from build123d import *

# Parameters (mm, degrees)
PAD_DEPTH       = 25
FILLET_R        = 3
SKETCH009_R     = 7
PAD001_DEPTH    = 6
SKETCH_R        = 12.5
PAD002_DEPTH    = 9.5
POCKET_DEPTH    = 21.498539
SKETCH003_R     = 2.9
POCKET001_DEPTH = 21.498539
POCKET002_DEPTH = 16
POCKET003_DEPTH = 27
SKETCH008_R     = 3.6
POCKET004_DEPTH = 10
SKETCH017_R     = 6.528292
POCKET005_DEPTH = 3
CHAMFER_SIZE    = 2


with BuildPart() as part:
    # Sketch007 → Pad (new body, symmetric)
    with BuildSketch(Plane.XY):
        Polygon((0, 0), (6, 0), (6, 33.225744), (20.888192, 31.397703), (21.497539, 36.360434), (0, 39), align=None)
    extrude(amount=PAD_DEPTH, both=True)

    # Fillet
    fillet_edges = [part.edges().sort_by_distance(p)[0] for p in [
        (0, 39, 0),
        (6, 33.225744, 0),
    ]]
    fillet(fillet_edges, radius=FILLET_R)

    # Sketch009 (on Face7 of Fillet) → Pad001 (join)
    with BuildSketch(Plane(origin=(0, 0, 0), x_dir=(0, -1, 0), z_dir=(-1, 0, 0))):
        with Locations((-7, 25)):
            Circle(SKETCH009_R)
    extrude(amount=-PAD001_DEPTH)

    # Sketch → Pad002 (join)
    with BuildSketch(Plane(origin=(0, 0, 0), x_dir=(0, -1, 0), z_dir=(-1, 0, 0))):
        with BuildLine():
            Line((40.112649, -31.334923), (0, -1.650119))
            Line((0, -1.650119), (-36.144043, -17.199829))
            Line((19.887351, -58.665077), (-36.144043, -17.199829))
            ThreePointArc((19.887351, -58.665077), (43.665077, -55.112649), (40.112649, -31.334923))
        make_face()
        with Locations((30, -45)):
            Circle(SKETCH_R, mode=Mode.SUBTRACT)
    extrude(amount=-PAD002_DEPTH)

    # Sketch013 → Pocket (cut, through all)
    with BuildSketch(Plane(origin=(0, 0, 0), x_dir=(0, -1, 0), z_dir=(-1, 0, 0))):
        Polygon((22.699889, -37.062297), (13.507356, -29.348846), (26.630219, -13.709626), (25.864174, -13.066839), (11.455736, -30.238147), (21.414314, -38.594386), align=None)
    extrude(amount=-POCKET_DEPTH, mode=Mode.SUBTRACT)

    # Sketch003 (on Face19 of Pad002) → Pocket001 (cut, through all)
    with BuildSketch(Plane(origin=(0, 0, 0), x_dir=(0, -1, 0), z_dir=(-1, 0, 0))):
        with Locations((-7, -25)):
            Circle(SKETCH003_R)
        with Locations((-7, 25)):
            Circle(SKETCH003_R)
    extrude(amount=-POCKET001_DEPTH, mode=Mode.SUBTRACT)

    # Sketch015 → Pocket002 (cut)
    with BuildSketch(Plane(origin=(0, 0.311228, -0.406819), x_dir=(1, 0, 0), z_dir=(0, -0.607611, 0.794235))):
        Polygon((4.690891, -37.115485), (6.690891, -35.960785), (6.690891, -33.651383), (4.690891, -32.496683), (2.690891, -33.651383), (2.690891, -35.960785), align=None)
    extrude(amount=-POCKET002_DEPTH, mode=Mode.SUBTRACT)

    # Sketch014 → Pocket003 (cut)
    with BuildSketch(Plane(origin=(0, 0.311228, -0.406819), x_dir=(1, 0, 0), z_dir=(0, -0.607611, 0.794235))):
        Polygon((6.15, -35.644522), (6.15, -34.027942), (4.75, -33.219651), (3.35, -34.027942), (3.35, -35.644522), (4.75, -36.452813), align=None)
    extrude(amount=-POCKET003_DEPTH, mode=Mode.SUBTRACT)

    # Sketch008 (on Face11 of Pocket003) → Pocket004 (cut)
    with BuildSketch(Plane(origin=(4.717477, 38.420767, 0), x_dir=(-0.992546, 0.121869, 0), z_dir=(0.121869, 0.992546, 0))):
        with Locations((-8, 0)):
            Circle(SKETCH008_R)
    extrude(amount=-POCKET004_DEPTH, mode=Mode.SUBTRACT)

    # Sketch017 (on Face7 of Pocket004) → Pocket005 (cut)
    with BuildSketch(Plane.YZ.offset(9.5)):
        with Locations((6.933498, -25.139439)):
            Circle(SKETCH017_R)
    extrude(amount=-POCKET005_DEPTH, mode=Mode.SUBTRACT)

    # Chamfer
    chamfer_edges = [part.edges().sort_by_distance(p)[0] for p in [
        (9.5, 0.405206, -25.139439),
    ]]
    chamfer(chamfer_edges, length=CHAMFER_SIZE)


solid = part.part
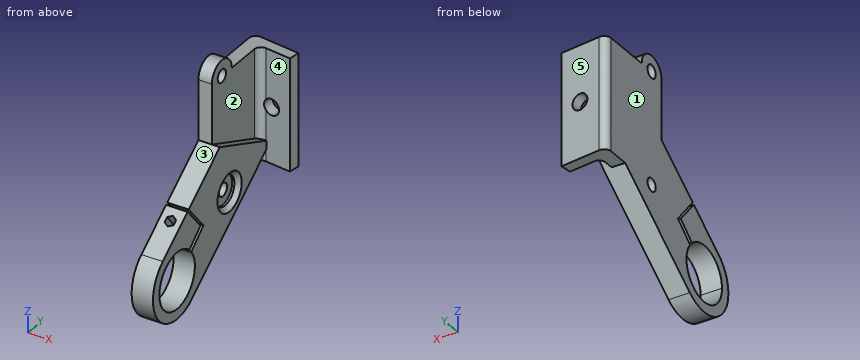
Could you check a few things on this model? Use its own coordinates, in mm. Face numbers are marked on the shaded views. A direction names the side the tool comes from. Give positions to 0.01 mm unless a question says otherwise; leave off trailing zeros. Order: outer loops, then holes, each group sorted by start corner. A loop starts at its lowest first (then second) coordinate and runs counter-clockwise, first axis right, second up.
1. For the marked faces 1 and 2, which set-ups out of +Z, -Z, +X, -X, +Y, -Y let a thin tool reach every point of the face, with its end or its side?
2. Will these pins go through, and if not, where does the flat tip stop? P1, Ø6.5, axis at x = 4, z = 6.5, coming from the -Y side; P2, Ø2, axis at x = 7.5, z = -18, coming from the +Y side; P3, Ø4, axis at y = 8, z = -24.5, coming from the +X side.
3. I need wall thicknesses on L1, parallel to Z at x = 1.4, y = 7; L2, parallel to Z at x = 3.25, y = 35; L3, parallel to X at y = -26.5, z = -22. Which ranges of each line are inside material? Lowest first, please.
4. Suppose I cut it at A-A (y = -35.5). List the corners of the cut face in (x, z) for me, plus the area to 3 significant figures.
5. Suppose I cut it at C-C (z = -5.5). List the corners of the cut face in (x, y) for me.
6. Suppose I cut it at D-D (y = -4.5). List the corners of the cut face in (x, z) for me.
7. Suppose I cut it at B-B (x = 1.5). List the corners of the cut face in (y, z) for me.
8. We'd pull the mould along X, two halves only. Please class the marked faces 3, 4 and 5: pulls with the +X half, pulls with the -X half, needs draft (parallel to the pull), parting line crosses it, or undercut.
Solved:
1. face 1: +Z, -Z, -X, +Y, -Y
1. face 2: +Z, +X
2. P1: stops at y = 0
2. P2: stops at y = 38.2
2. P3: stops at x = 6.5
3. L1: z = -38.77 to -27.9, -22.1 to 22.1, 27.9 to 32
3. L2: z = -25 to 25
3. L3: x = 0 to 2.69, 6.69 to 9.5
4. outline: (0, -61.09) - (9.5, -61.09) - (9.5, -56.22) - (0, -56.22) - close; (0, -33.78) - (9.5, -33.78) - (9.5, -27.92) - (0, -27.92) - close
4. area: 102 mm2
5. outline: (0, -5.2) - (9.5, -5.2) - (9.5, 8.95) - (6, 8.95) - (6, 29.83) arc R3 cw to (9.37, 32.81) - (20.89, 31.4) - (21.5, 36.36) - (3.37, 38.59) arc R3 ccw to (0, 35.61) - close
6. outline: (0, -47.28) - (9.5, -47.28) - (9.5, -4.98) - (0, -4.98) - close
7. outline: (-40.11, -31.33) arc R17 ccw to (-19.89, -58.67) - (25.6, -25) - (38.21, -25) - (38.21, 25) - (14, 25) arc R7 ccw to (0, 25) - (0, -1.65) - (-21.87, -17.83) - (-11.46, -30.24) - (-20.04, -37.44) arc R12.5 cw (long way) to (-21.38, -35.95) - (-13.51, -29.35) - (-22.67, -18.43) - close; hole circle Ø5.8 at (7, -25); hole circle Ø5.8 at (7, 25)
8. face 3: needs draft
8. face 4: undercut
8. face 5: pulls with the +X half
